```python
from build123d import *

# Parameters (mm, degrees)
BOSS_EXTRUDE5_DEPTH = 23
SKETCH3_W           = 5
SKETCH3_H           = 3
BOSS_EXTRUDE7_DEPTH = 42.2
CUT_EXTRUDE3_DEPTH  = 42.2
CUT_EXTRUDE4_DEPTH  = 42.2
FILLET1_R           = 3
FILLET2_R           = 3
FILLET3_R           = 0.5
FILLET4_R           = 0.5
FILLET5_R           = 3
FILLET6_R           = 3
CUT_EXTRUDE5_DEPTH  = 42.2
CUT_EXTRUDE6_DEPTH  = 42.2
CUT_EXTRUDE7_DEPTH  = 42.2


with BuildPart() as part:
    # Sketch1 → Boss-Extrude5 (new body)
    with BuildSketch(Plane(origin=(0, 0, 0), x_dir=(1, 0, 0), z_dir=(0, 1, 0))):
        Polygon((-55, 0), (55, 0), (55, 3), (26.1, 3), (26.1, 45.2), (21.1, 45.2), (21.1, 3), (-21.1, 3), (-21.1, 45.2), (-26.1, 45.2), (-26.1, 3), (-55, 3), align=None)
    extrude(amount=BOSS_EXTRUDE5_DEPTH)

    # Sketch3 → Boss-Extrude7 (add)
    with BuildSketch(Plane(origin=(0, 0, -3), x_dir=(-1, 0, 0), z_dir=(0, 0, -1))):
        with Locations((-18.6, 21.5)):
            Rectangle(SKETCH3_W, SKETCH3_H)
        with Locations((18.6, 21.5)):
            Rectangle(SKETCH3_W, SKETCH3_H)
    extrude(amount=BOSS_EXTRUDE7_DEPTH)

    # Sketch5 → Cut-Extrude3 (cut)
    with BuildSketch(Plane(origin=(0, 20, 0), x_dir=(-1, 0, 0), z_dir=(0, -1, 0))):
        with BuildLine():
            Line((-17.6, 43.490720045), (-17.6, 4.709279955))
            ThreePointArc((-17.6, 4.709279955), (-18.6, 3.709279955), (-19.6, 4.709279955))
            Line((-19.6, 4.709279955), (-19.6, 43.490720045))
            ThreePointArc((-19.6, 43.490720045), (-18.6, 44.490720045), (-17.6, 43.490720045))
        make_face()
    extrude(amount=-CUT_EXTRUDE3_DEPTH, mode=Mode.SUBTRACT)

    # Sketch5<4> → Cut-Extrude4 (cut)
    with BuildSketch(Plane(origin=(0, 20, 0), x_dir=(-1, 0, 0), z_dir=(0, -1, 0))):
        with BuildLine():
            Line((17.6, 4.709279955), (17.6, 43.490720045))
            ThreePointArc((17.6, 43.490720045), (18.6, 44.490720045), (19.6, 43.490720045))
            Line((19.6, 43.490720045), (19.6, 4.709279955))
            ThreePointArc((19.6, 4.709279955), (18.6, 3.709279955), (17.6, 4.709279955))
        make_face()
    extrude(amount=-CUT_EXTRUDE4_DEPTH, mode=Mode.SUBTRACT)

    # Fillet1
    fillet1_edges = [part.edges().sort_by_distance(p)[0] for p in [
        (-26.1, 11.5, -45.2),
    ]]
    fillet(fillet1_edges, radius=FILLET1_R)

    # Fillet2
    fillet2_edges = [part.edges().sort_by_distance(p)[0] for p in [
        (26.1, 11.5, -45.2),
    ]]
    fillet(fillet2_edges, radius=FILLET2_R)

    # Fillet3
    fillet3_edges = [part.edges().sort_by_distance(p)[0] for p in [
        (-16.1, 21.5, -45.2),
    ]]
    fillet(fillet3_edges, radius=FILLET3_R)

    # Fillet4
    fillet4_edges = [part.edges().sort_by_distance(p)[0] for p in [
        (16.1, 21.5, -45.2),
    ]]
    fillet(fillet4_edges, radius=FILLET4_R)

    # Fillet5
    fillet5_edges = [part.edges().sort_by_distance(p)[0] for p in [
        (55, 11.5, -3),
    ]]
    fillet(fillet5_edges, radius=FILLET5_R - 0.0001)  # a hair under: the kernel refuses the full size

    # Fillet6
    fillet6_edges = [part.edges().sort_by_distance(p)[0] for p in [
        (-55, 11.5, -3),
    ]]
    fillet(fillet6_edges, radius=FILLET6_R - 0.0001)  # a hair under: the kernel refuses the full size

    # Sketch6 → Cut-Extrude5 (cut)
    with BuildSketch(Plane(origin=(0, 0, -3), x_dir=(-1, 0, 0), z_dir=(0, 0, -1))):
        with BuildLine():
            Line((-29.05, 15.25), (-49.05, 15.25))
            ThreePointArc((-49.05, 15.25), (-51.05, 17.25), (-49.05, 19.25))
            Line((-49.05, 19.25), (-29.05, 19.25))
            ThreePointArc((-29.05, 19.25), (-27.05, 17.25), (-29.05, 15.25))
        make_face()
        with BuildLine():
            Line((-29.05, 3.75), (-49.05, 3.75))
            ThreePointArc((-49.05, 3.75), (-51.05, 5.75), (-49.05, 7.75))
            Line((-49.05, 7.75), (-29.05, 7.75))
            ThreePointArc((-29.05, 7.75), (-27.05, 5.75), (-29.05, 3.75))
        make_face()
    extrude(amount=-CUT_EXTRUDE5_DEPTH, mode=Mode.SUBTRACT)

    # Sketch7 → Cut-Extrude6 (cut)
    with BuildSketch(Plane(origin=(0, 0, -3), x_dir=(-1, 0, 0), z_dir=(0, 0, -1))):
        with BuildLine():
            Line((49.05, 15.25), (29.05, 15.25))
            ThreePointArc((29.05, 15.25), (27.05, 17.25), (29.05, 19.25))
            Line((29.05, 19.25), (49.05, 19.25))
            ThreePointArc((49.05, 19.25), (51.05, 17.25), (49.05, 15.25))
        make_face()
    extrude(amount=-CUT_EXTRUDE6_DEPTH, mode=Mode.SUBTRACT)

    # Sketch7<3> → Cut-Extrude7 (cut)
    with BuildSketch(Plane(origin=(0, 0, -3), x_dir=(-1, 0, 0), z_dir=(0, 0, -1))):
        with BuildLine():
            Line((29.05, 7.503040911), (49.05, 7.503040911))
            ThreePointArc((49.05, 7.503040911), (51.05, 5.503040911), (49.05, 3.503040911))
            Line((49.05, 3.503040911), (29.05, 3.503040911))
            ThreePointArc((29.05, 3.503040911), (27.05, 5.503040911), (29.05, 7.503040911))
        make_face()
    extrude(amount=-CUT_EXTRUDE7_DEPTH, mode=Mode.SUBTRACT)


solid = part.part
```
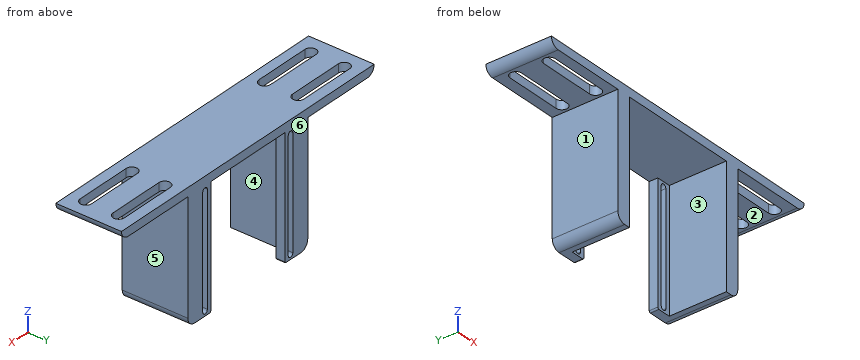
Part model, mm, in its own coordinate system. Face numbers are marked on the shaded views. A direction names the side the tool comes from. Round coordinates to 2 decimals unless told otherwise and drop trailing zeros. Loops run counter-clockwise (first coordinate to the right, second up) from the corner with the lowest first, then second, coordinate; pieces in that order, holes last.
Item 1: Drop flat-ended pins along their axis: P1, Ø0.9, axis at x = 40, z = -1.5, coming from the -Y side; P2, Ø1, axis at x = 5, y = 4, coming from the -Z side; P3, Ø1.5, axis at y = 13, z = -30, coming from the -X side; P4, Ø1.5, axis at y = 22, z = -27, coming from the +X side. Give the stop position or say it passes through.
Item 2: Cut at B-B, the plane x = -36. Give the cut face in (y, z).
Item 3: Mould opens along X. For the marked faces 4, 5 and 6 say: +X half, -X half, draft (parallel to the pull), parting line (faces both ways), or undercut.
Item 4: Cut at A-A, the plane z = -22.5. Give the cut face in (x, y), then the cut area to 3 significant figures.
Item 5: Cut at D-D, the plane x = 18.6. Give the cut face in (y, z), then the cut area to 3 significant figures.
Item 6: 3-axis set-ups, long thin cutter, end or side, ignore diameter. For the marked faces 1, 2 and 3: which of +Z, -Z, +X, -X, +Y, -Y reach the whole face in a straight line?
Item 7: Cut at C-C, the plane y = 17.25. State how many separate pieces and enclosed holes the cut face has, then the cut area to 3 significant figures.
Item 8: Drill centre lines: line 1 (X direction, y = 10.25, z = -31); line 2 (Z direction, x = 15, y = 22.25); line 3 (X direction, y = 2, z = -2). Where is each one in solid material? Low to high.
A:
1. P1: stops at y = 0
1. P2: stops at z = -3
1. P3: stops at x = -26.1
1. P4: stops at x = 26.1
2. outline: (0, -3) - (3.5, -3) - (3.5, 0) - (0, 0) - close; (7.5, -3) - (15.25, -3) - (15.25, 0) - (7.5, 0) - close; (19.25, -3) - (23, -3) - (23, 0) - (19.25, 0) - close
3. face 4: undercut
3. face 5: +X half
3. face 6: draft
4. outline: (-26.1, 0) - (-21.1, 0) - (-21.1, 20) - (-19.6, 20) - (-19.6, 23) - (-26.1, 23) - close; (-17.6, 20) - (-16.1, 20) - (-16.1, 23) - (-17.6, 23) - close; (16.1, 20) - (17.6, 20) - (17.6, 23) - (16.1, 23) - close; (19.6, 20) - (21.1, 20) - (21.1, 0) - (26.1, 0) - (26.1, 23) - (19.6, 23) - close
4. area: 248 mm2
5. outline: (0, -3) - (20, -3) - (20, -3.71) - (23, -3.71) - (23, 0) - (0, 0) - close; (20, -45.2) - (23, -45.2) - (23, -44.49) - (20, -44.49) - close
5. area: 73.3 mm2
6. face 1: -Z, -X, +Y, -Y
6. face 2: -Z, +X, +Y, -Y
6. face 3: -Z, -Y
7. separate pieces: 3
7. enclosed holes: 0
7. area: 600 mm2
8. line 1: x = -26.1 to -21.1, 21.1 to 26.1
8. line 2: z = -3 to 0
8. line 3: x = -54.24 to 54.24
